Model file for the job. Use its own axes, mm. A direction names the side the tool comes from. Coordinates: 2 decimals unless noted, no trailing zeros. Order: outer loops, then holes, each group sorted by start corner. A loop starts at its lowest first (then second) coordinate and runs counter-clockwise, first axis right, second up. Notation, with made-up numbers: (-39, 22) -> (-7, 22) arc R13 cw to (-7, 31) -> close; hole circle Ø9 at (34, -19). An arc over 180 degrees is marked (long way). Return JSON: item names as keys, results as strings. Group by question number.
1) Cut at B-B (y = 1.5). Write the cut outline in (x, z).
2) Pull direction X, two halves, no side cores. Call faces 1 (the cylindrical face through (72.231, -1.777, -0.018)), 2 (the flat face through (-1, -17.78, 0)), 3 (the flat face through (80.607, 0, 0)), 4 (the flat face through (65.033, 0, 0)): +X half, -X half, draft (parallel to the pull), parting line (faces both ways), or undercut.
3) Cut at A-A (x = 15.5). Write the cut outline in (y, z).
4) Cut at C-C (z = -0.2). Write the cut outline in (x, y), and give its area (3 significant figures).
5) Which spindle directions (+Z, -Z, +X, -X, +Y, -Y) get a long thin tool onto all of the face, cutting with end or side? Do faces 5 (the flat face through (-1, 7.62, 0)), 6 (the flat face through (-1, 8, -1.27)). Say none if no direction does.
6) Probe line 1 (X direction, y = -8.5, z = 1.15); line 2 (Y direction, x = -34, z = 0); line 3 (X direction, y = 1, z = 0). List the from-to ranges inside material, lowest first.
from build123d import *

# Parameters (mm, degrees)
F0_R     = 2.921
F0_W     = 131.063283
F0_H     = 15.24
F1_DEPTH = 1.27


with BuildPart() as f1:
    # F0 (on Top) → F1 (new body, symmetric)
    with BuildSketch(Plane.XY):
        Polygon((80.6069, -17.78), (80.6069, 17.78), (68.4911, 17.78), (-68.4911, 17.78), (-80.6069, 17.78), (-80.6069, -17.78), (-68.4911, -17.78), (68.4911, -17.78), align=None)
        with Locations((-74.549, -8.89)):
            Circle(F0_R, mode=Mode.SUBTRACT)
        with Locations((-74.549, 0)):
            Circle(F0_R, mode=Mode.SUBTRACT)
        with Locations((-0.498816, 0)):
            Rectangle(F0_W, F0_H, mode=Mode.SUBTRACT)
        with Locations((74.549, -8.89)):
            Circle(F0_R, mode=Mode.SUBTRACT)
        with Locations((74.549, 0)):
            Circle(F0_R, mode=Mode.SUBTRACT)
        with Locations((-74.549, 8.89)):
            Circle(F0_R, mode=Mode.SUBTRACT)
        with Locations((74.549, 8.89)):
            Circle(F0_R, mode=Mode.SUBTRACT)
    extrude(amount=F1_DEPTH, both=True)


solid = f1.part
Answers below:
{
 "1": {"outline": "(-80.61, -1.27) -> (-77.06, -1.27) -> (-77.06, 1.27) -> (-80.61, 1.27) -> close; (-72.04, -1.27) -> (-66.03, -1.27) -> (-66.03, 1.27) -> (-72.04, 1.27) -> close; (65.03, -1.27) -> (72.04, -1.27) -> (72.04, 1.27) -> (65.03, 1.27) -> close; (77.06, -1.27) -> (80.61, -1.27) -> (80.61, 1.27) -> (77.06, 1.27) -> close"},
 "2": {"face 1": "undercut", "face 2": "draft", "face 3": "+X half", "face 4": "undercut"},
 "3": {"outline": "(-17.78, -1.27) -> (-7.62, -1.27) -> (-7.62, 1.27) -> (-17.78, 1.27) -> close; (7.62, -1.27) -> (17.78, -1.27) -> (17.78, 1.27) -> (7.62, 1.27) -> close"},
 "4": {"outline": "(-80.61, -17.78) -> (80.61, -17.78) -> (80.61, 17.78) -> (-80.61, 17.78) -> close; hole circle Ø5.84 at (-74.55, -8.89); hole circle Ø5.84 at (-74.55, 0); hole circle Ø5.84 at (-74.55, 8.89); hole (-66.03, -7.62) -> (65.03, -7.62) -> (65.03, 7.62) -> (-66.03, 7.62) -> close; hole circle Ø5.84 at (74.55, -8.89); hole circle Ø5.84 at (74.55, 0); hole circle Ø5.84 at (74.55, 8.89)", "area": "3,570 mm^2"},
 "5": {"face 5": "+Z, -Z", "face 6": "-Z, +X, -X, +Y, -Y"},
 "6": {"line 1": "x = -80.61 to -77.44, -71.65 to 71.65, 77.44 to 80.61", "line 2": "y = -17.78 to -7.62, 7.62 to 17.78", "line 3": "x = -80.61 to -77.29, -71.8 to -66.03, 65.03 to 71.8, 77.29 to 80.61"}
}
